Input: part model. Units: mm. Frame: model coordinates. A direction names the side the tool comes from. Coordinates: 2 decimals unless noted, no trailing zeros. Order: outer loops, then holes, each group sorted by start corner. A loop starts at its lowest first (then second) coordinate and runs counter-clockwise, first axis right, second up. Notation, with made-up numbers: (-10.5, 31.5) -> (11.5, 31.5) arc R13 cw to (11.5, 43.5) -> close; hole circle Ø3 at (54.25, 47.5). An arc over 180 degrees is marked (long way). Use one line per item in the form item = value. Start each with the question number.
1) Access query for faces 1 (the flat face through (2, 0.5, 80)), 2 (the flat face through (0, 0, -130)). Directions: +Z, -Z, +X, -X, +Y, -Y. A direction counts if a zero-diameter tool reaches every point of the face in a straight line with its end or side. Return the directions, or none.
2) Section query A-A on z = 0. Output: boundary loops of the cut face in (x, y).
3) Ray query, line 1 along X through (y, z) = (4, 40); line 2 along X through (y, z) = (-2.65, 120); line 3 along Y through (x, z) = (7.25, -105.5). Return the intervals inside material, ascending.
4) Draft query along X for faces 3 (the flat face through (7.5, -2, -2)), 4 (the cylindrical face through (-0.9, 2.72, -117.14)), 5 (the flat face through (3, -5, -2)), 6 (the cylindrical face through (0, 3, 37)). Return one class per face: pulls with the +X half, pulls with the -X half, needs draft (parallel to the pull), parting line crosses it, or undercut.
5) Section query B-B on z = -53. Output: boundary loops of the cut face in (x, y), then the cut area to 3 significant figures.
6) Pin query (flat end, axial travel): pin 1 (3 mm diameter, centred on x = 0, z = -40, fed in from -Y); pin 2 (3 mm diameter, centred on x = -0.5, z = -39.5, fed in from +Y). Return the tip coordinate at first contact, or that it passes through.
Autodesk Inventor part; units mm, degrees
ref_plane "YZ Plane" through (0, 0, 0) normal (1, 0, 0) x (0, 1, 0)
ref_plane "XZ Plane" through (0, 0, 0) normal (0, 1, 0) x (-1, 0, 0)
ref_plane "XY Plane" through (0, 0, 0) normal (0, 0, 1) x (1, 0, 0)
sketch "Sketch1" plane through (0, 0, 0) normal (0, 0, 1) x (1, 0, 0)
  line L0 (-7.5, 5) -> (7.5, 5)
  line L1 (7.5, 5) -> (7.5, -5)
  line L2 (7.5, -5) -> (-7.5, -5)
  line L3 (-7.5, -5) -> (-7.5, 5)
  line L4 (-7.5, 5) -> (7.5, -5) construction
  line L5 (7.5, 5) -> (-7.5, -5) construction
  line L6 (-7.5, 3.0607) -> (-6.4393, 2)
  line L7 (-7.5, 3.0607) -> (-6, 3.0607) construction
  line L8 (-6.4393, 2) -> (-7.5, 0.9393)
  line L9 (0, 5) -> (0, -5) construction
  line L10 (7.5, 3.0607) -> (6.4393, 2)
  line L11 (6.4393, 2) -> (7.5, 0.9393)
  point P0 (0, 0)
  point P1 (7.5, 0.9393)
  point P2 (7.5, 3.0607)
  dimension "d0" = 15
  dimension "d1" = 10
  dimension "d2" = 45
  dimension "d3" = 3
  dimension "d4" = 1.5
extrude "Extrusion1" add sketch "Sketch1" along normal mid plane 260 contours L0 L1 L10 L11 L2 L3 L8 L6
sketch "Sketch2" plane through (-7.5, 5, 130) normal (0, 1, 0) x (1, 0, 0)
  point P0 (7.5, 130)
  point P1 (7.5, 130)
hole "Hole1" at (0, 5, 0) direction (0, -1, 0) diameter 3.5 end through all counterbore diameter 6 counterbore depth 4.5
pattern_linear "Rectangular Pattern1" count 9 spacing 40 along (0, 0, 1) of "Hole1" first direction both ways yes
sketch "Sketch3" plane through (-7.5, 5, 130) normal (0, 1, 0) x (1, 0, 0)
  point P0 (7.5, 130)
  point P1 (7.5, 130)
hole "Hole2" at (0, 5, 0) direction (0, -1, 0) diameter 6 end through all
properties part number "MGN15 Rail" material "Stainless Steel, 440C"
Answers below:
q1.face_1 = +Y
q1.face_2 = -Z, +X, -X, +Y, -Y
q2.outline = (-7.5, -5) -> (-3, -5) -> (-3, 5) -> (-7.5, 5) -> (-7.5, 3.06) -> (-6.44, 2) -> (-7.5, 0.94) -> close; (3, -5) -> (7.5, -5) -> (7.5, 0.94) -> (6.44, 2) -> (7.5, 3.06) -> (7.5, 5) -> (3, 5) -> close
q3.line_1 = -7.5 to -3, 3 to 7.5
q3.line_2 = -7.5 to -1.75, 1.75 to 7.5
q3.line_3 = -5 to 1.19, 2.81 to 5
q4.face_3 = pulls with the +X half
q4.face_4 = undercut
q4.face_5 = needs draft
q4.face_6 = undercut
q5.outline = (-7.5, -5) -> (7.5, -5) -> (7.5, 0.94) -> (6.44, 2) -> (7.5, 3.06) -> (7.5, 5) -> (-7.5, 5) -> (-7.5, 3.06) -> (-6.44, 2) -> (-7.5, 0.94) -> close
q5.area = 148 mm^2
q6.pin_1 = through
q6.pin_2 = 0.5
